Answer from the drawing. Dimensions are ordinates in mm from the lowest x, y and z of the part. A direction names the side the tool comes from. Coordinates: 2 decimals unless noted, no trailing zeros. Write each loop counter-clockwise with the first axis right and the second up, starting at its lowest first coordinate (ties: lowest second). Pieces come first, ordered by that corner, then holes. Notation, with made-up numbers: (-25, 1.25) - (26, 1.25) arc R31 cw to (26, 26.25) - close; hole circle Ø2 at (78, -24.5). An arc over 180 degrees is marked (long way). Use a Markdown table: item, result.
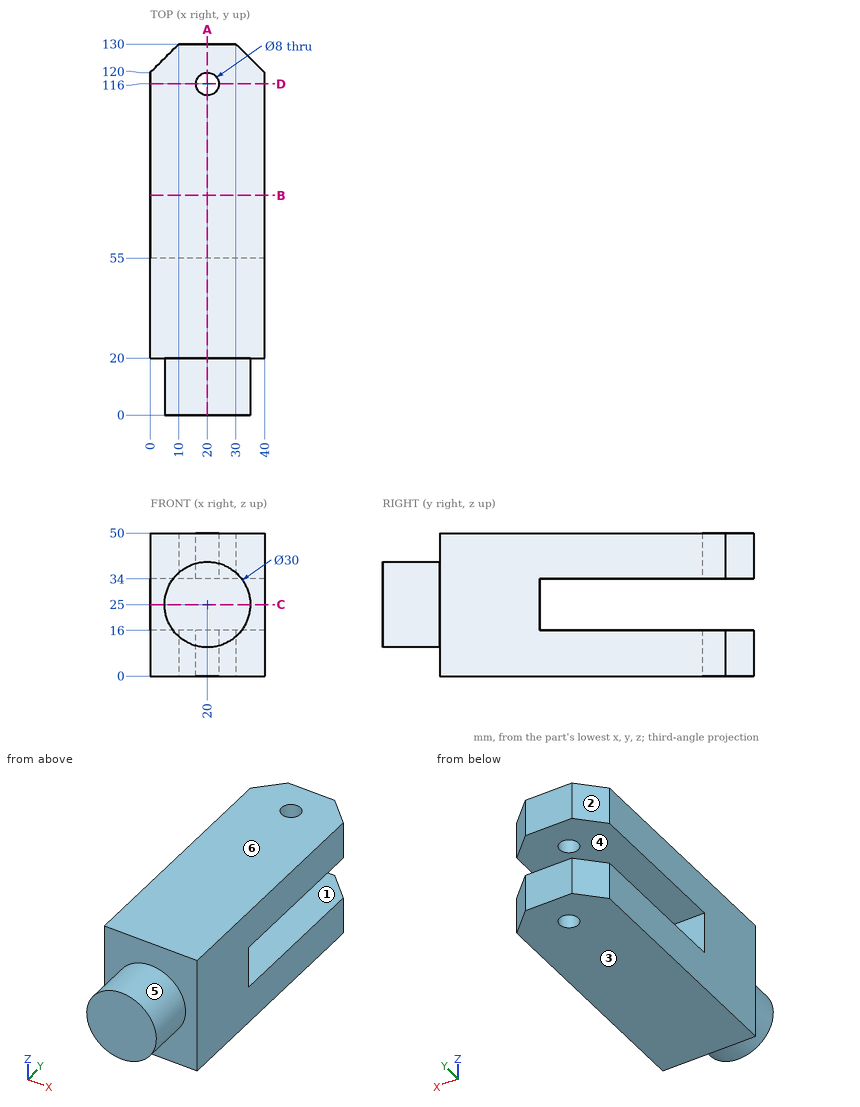
(1) Each of these flat-tipped pins is pushed along its axis until it touches: P1, Ø8, axis at x = 22.5, y = 19.5, coming from the +Z side; P2, Ø6.5, axis at x = 20, y = 116, coming from the -Z side; P3, Ø5, axis at x = 36, z = 26, coming from the +Y side; P4, Ø3, axis at x = 6.5, z = 39.5, coming from the -Y side. Where does it stop, or does it pass through?
Report:
| item | result |
|---|---|
| P1 | stops at z = 50 |
| P2 | passes through |
| P3 | stops at y = 55 |
| P4 | stops at y = 20 |
(2) The mould has two halves that part along Z. Classify the marked faces 1, 2 and 3: pulls with the +Z half, pulls with the -Z half, needs draft (parallel to the pull), parting line crosses it, or undercut.
Report:
| item | result |
|---|---|
| face 1 | undercut |
| face 2 | needs draft |
| face 3 | pulls with the -Z half |
(3) For the marked faces 4, 5 and 6, determine the directions among +Z, -Z, +X, -X, +Y, -Y from which every point of the face is accessible in a straight line to the end or side of a thin tool.
Report:
| item | result |
|---|---|
| face 4 | +X, -X, +Y |
| face 5 | -Y |
| face 6 | +Z, +X, -X, +Y, -Y |
(4) A cutting plane is placed at C-C, the plane z = 25. Write down the section's boundary in (x, y).
Report:
| item | result |
|---|---|
| outline | (0, 20) - (5, 20) - (5, 0) - (35, 0) - (35, 20) - (40, 20) - (40, 55) - (0, 55) - close |
(5) Straight lines are drawn through the part: L1, parallel to Y at x = 20, z = 43.25; L2, parallel to Y at x = 20, z = 12.5; L3, parallel to Z at x = 9.5, y = 109. For each, find the intervals that lie inside material, in ascending order.
Report:
| item | result |
|---|---|
| L1 | y = 20 to 112, 120 to 130 |
| L2 | y = 0 to 112, 120 to 130 |
| L3 | z = 0 to 16, 34 to 50 |
(6) A cutting plane is placed at A-A, the plane x = 20. Write down the section's boundary in (y, z), and give its area (3 significant figures).
Report:
| item | result |
|---|---|
| outline | (0, 10) - (20, 10) - (20, 0) - (112, 0) - (112, 16) - (55, 16) - (55, 34) - (112, 34) - (112, 50) - (20, 50) - (20, 40) - (0, 40) - close; (120, 0) - (130, 0) - (130, 16) - (120, 16) - close; (120, 34) - (130, 34) - (130, 50) - (120, 50) - close |
| area | 4,490 mm² |
(7) A cutting plane is placed at B-B, the plane y = 77. Write down the section's boundary in (x, z).
Report:
| item | result |
|---|---|
| outline | (0, 0) - (40, 0) - (40, 16) - (0, 16) - close; (0, 34) - (40, 34) - (40, 50) - (0, 50) - close |
(8) A cutting plane is placed at D-D, the plane y = 116. Write down the section's boundary in (x, z).
Report:
| item | result |
|---|---|
| outline | (0, 0) - (16, 0) - (16, 16) - (0, 16) - close; (0, 34) - (16, 34) - (16, 50) - (0, 50) - close; (24, 0) - (40, 0) - (40, 16) - (24, 16) - close; (24, 34) - (40, 34) - (40, 50) - (24, 50) - close |
